Read the model definition and answer for the solid it produces. Units are mm, in the model's axes. A direction names the side the tool comes from. Coordinates: 2 decimals unless noted, no trailing zeros. Loops run counter-clockwise (first coordinate to the right, second up) from the corner with the lowest first, then second, coordinate; pieces in that order, holes last. Notation, with made-up numbers: (51.25, -17) -> (57.25, -17) arc R28 ccw to (57.25, 9) -> close; hole circle Ø1 at (25.5, 11.5). An arc over 180 degrees is marked (long way). Answer as a JSON object with one key per item and string values. Group by question number.
Q1. Each of these flat-tipped pins is pushed along its axis until it touches: P1, Ø4.5, axis at y = -25, z = 48, coming from the -X side; P2, Ø1.9, axis at y = -25, z = 12.5, coming from the +X side; P3, Ø0.8, axis at y = -27, z = 83.5, coming from the -X side; P4, Ø4, axis at x = -14, y = -20.5, coming from the -Z side. Where does it stop, or does it pass through?
Q2. The part is cut by section C-C on x = 40.5. Write down the section's boundary in (y, z).
Q3. Determine the mould class of faces 4 (the flat face through (-10, -24, 70)), 5 (the flat face through (36, -27.495, 49)), 6 (the flat face through (-7, -25, 100)) for opening direction Z: released by +Z, released by -Z, zero draft, split by the parting line, or undercut.
Q4. The part is cut by section B-B on z = 67.5. Write down the section's boundary in (x, y), and give its area (3 significant figures).
Q5. The part is cut by section A-A on x = -2.5. Write down the section's boundary in (y, z), and give its area (3 significant figures).
Q6. Straight lines are drawn through the part: line 1 along Z through (x, y) = (-22.5, -21.75); line 2 along X through (y, z) = (-25.25, 13); line 3 along Y through (x, z) = (44.5, 78). For each, find the intervals that lie inside material, in ascending order. Write a range as [from, to].
Q7. The part is cut by section D-D on z = 38.5. Write down the section's boundary in (x, y), and give its area (3 significant figures).
Q8. For faces 1 (the flat face through (-9, -24, 30)), 2 (the flat face through (-7, -25, 0)), 3 (the flat face through (4.258, -26, 85)), determine the directions among +Z, -Z, +X, -X, +Y, -Y from which every point of the face is accessible in a straight line to the end or side of a thin tool.
from build123d import *

# Parameters (mm, degrees)
BOSS_EXTRUDE1_DEPTH     = 100
CUT_EXTRUDE1_DEPTH      = 24
CUT_EXTRUDE1_DEPTH_BACK = 24
FILLET2_R               = 25
SKETCH4_W               = 13
SKETCH4_H               = 10
CUT_EXTRUDE3_DEPTH      = 23


with BuildPart() as part:
    # Sketch1 → Boss-Extrude1 (new body)
    with BuildSketch(Plane.XY):
        with BuildLine():
            Line((-25.742274507, -27.495485701), (-25.742274507, -25.803839777))
            ThreePointArc((-25.742274507, -25.803839777), (-25.800853151, -25.66241842), (-25.942274507, -25.603839777))
            Line((-25.942274507, -25.603839777), (-26.659431795, -25.603839777))
            ThreePointArc((-26.659431795, -25.603839777), (-26.735968481, -25.588615683), (-26.800853151, -25.545261133))
            Line((-26.800853151, -25.545261133), (-27.683698081, -24.662416203))
            ThreePointArc((-27.683698081, -24.662416203), (-27.72705275, -24.597531247), (-27.742276725, -24.520994228))
            Line((-27.742276725, -24.520994228), (-27.742274507, -23.803840395))
            ThreePointArc((-27.742274507, -23.803840395), (-27.800852932, -23.662418639), (-27.942274507, -23.603839777))
            Line((-27.942274507, -23.603839777), (-28.659430376, -23.603840885))
            ThreePointArc((-28.659430376, -23.603840885), (-28.735967229, -23.588616851), (-28.800852042, -23.545262242))
            Line((-28.800852042, -23.545262242), (-29.683696972, -22.662417311))
            ThreePointArc((-29.683696972, -22.662417311), (-29.727051582, -22.597532499), (-29.742275616, -22.520995646))
            Line((-29.742275616, -22.520995646), (-29.742274507, -21.803839777))
            ThreePointArc((-29.742274507, -21.803839777), (-29.800853256, -21.662418316), (-29.942274803, -21.603839777))
            Line((-29.942274803, -21.603839777), (-30.659430376, -21.603840885))
            ThreePointArc((-30.659430376, -21.603840885), (-30.735967229, -21.588616851), (-30.800852042, -21.545262242))
            Line((-30.800852042, -21.545262242), (-31.683696972, -20.662417311))
            ThreePointArc((-31.683696972, -20.662417311), (-31.727051582, -20.597532499), (-31.742275616, -20.520995646))
            Line((-31.742275616, -20.520995646), (-31.742274507, -19.80383981))
            ThreePointArc((-31.742274507, -19.80383981), (-31.800854095, -19.662417476), (-31.942277212, -19.603839777))
            Line((-31.942277212, -19.603839777), (-32.659432785, -19.603840885))
            ThreePointArc((-32.659432785, -19.603840885), (-32.735969638, -19.588616851), (-32.80085445, -19.545262242))
            Line((-32.80085445, -19.545262242), (-33.683699381, -18.662417311))
            ThreePointArc((-33.683699381, -18.662417311), (-33.727054119, -18.597532189), (-33.742278024, -18.520994974))
            Line((-33.742278024, -18.520994974), (-33.742274507, -17.803842952))
            ThreePointArc((-33.742274507, -17.803842952), (-33.683696986, -17.662419543), (-33.542274507, -17.603839777))
            Line((-33.542274507, -17.603839777), (-23.942274507, -17.603839777))
            ThreePointArc((-23.942274507, -17.603839777), (-23.800853151, -17.66241842), (-23.742274507, -17.803839777))
            Line((-23.742274507, -17.803839777), (-23.742274507, -18.520997064))
            ThreePointArc((-23.742274507, -18.520997064), (-23.727050414, -18.597533751), (-23.683695863, -18.66241842))
            Line((-23.683695863, -18.66241842), (-22.800853151, -19.545261133))
            ThreePointArc((-22.800853151, -19.545261133), (-22.735968481, -19.588615683), (-22.659431795, -19.603839777))
            Line((-22.659431795, -19.603839777), (-21.942274507, -19.603839777))
            ThreePointArc((-21.942274507, -19.603839777), (-21.800853151, -19.66241842), (-21.742274507, -19.803839777))
            Line((-21.742274507, -19.803839777), (-21.742274507, -20.520997064))
            ThreePointArc((-21.742274507, -20.520997064), (-21.727050414, -20.597533751), (-21.683695863, -20.66241842))
            Line((-21.683695863, -20.66241842), (-20.800853151, -21.545261133))
            ThreePointArc((-20.800853151, -21.545261133), (-20.735968481, -21.588615683), (-20.659431795, -21.603839777))
            Line((-20.659431795, -21.603839777), (-19.942274507, -21.603839777))
            ThreePointArc((-19.942274507, -21.603839777), (-19.800853151, -21.66241842), (-19.742274507, -21.803839777))
            Line((-19.742274507, -21.803839777), (-19.742274507, -22.520997064))
            ThreePointArc((-19.742274507, -22.520997064), (-19.727050414, -22.597533751), (-19.683695863, -22.66241842))
            Line((-19.683695863, -22.66241842), (-18.742274507, -23.603839777))
            Line((-18.742274507, -23.603839777), (-17.742274507, -23.603839777))
            Line((-17.742274507, -23.603839777), (59.257725493, -23.603839777))
            Line((59.257725493, -23.603839777), (59.257725493, -27.495485701))
            Line((59.257725493, -27.495485701), (-25.742274507, -27.495485701))
        make_face()
    extrude(amount=BOSS_EXTRUDE1_DEPTH)

    # Sketch2 → Cut-Extrude1 (cut, two sides: drawn at the far end of the back side and taken through both)
    with BuildSketch(Plane(origin=(0, -23.603839777, 0), x_dir=(1, 0, 0), z_dir=(0, 1, 0)).offset(-CUT_EXTRUDE1_DEPTH_BACK)):
        with BuildLine():
            Line((14.257725493, -30), (-42.622702361, -30))
            Line((-42.622702361, -30), (-42.622702361, -70))
            Line((-42.622702361, -70), (14.257725493, -70))
            ThreePointArc((14.257725493, -70), (24.864327211, -65.606601718), (29.257725493, -55))
            Line((29.257725493, -55), (29.257725493, -45))
            ThreePointArc((29.257725493, -45), (24.864327211, -34.393398282), (14.257725493, -30))
        make_face()
    extrude(amount=CUT_EXTRUDE1_DEPTH + CUT_EXTRUDE1_DEPTH_BACK, mode=Mode.SUBTRACT)

    # Fillet2
    fillet2_edges = [part.edges().sort_by_distance(p)[0] for p in [
        (59.257725493, -25.549662739, 100),
        (59.257725493, -25.549662739, 0),
    ]]
    fillet(fillet2_edges, radius=FILLET2_R)

    # Sketch4 → Cut-Extrude3 (cut)
    with BuildSketch(Plane(origin=(0, -23.603839777, 0), x_dir=(1, 0, 0), z_dir=(0, 1, 0))):
        with BuildLine():
            Line((14.257725493, -90), (14.257725493, -80))
            ThreePointArc((14.257725493, -80), (31.935395023, -72.67766953), (39.257725493, -55))
            Line((39.257725493, -55), (49.257725493, -55))
            ThreePointArc((49.257725493, -55), (39.006462834, -79.748737342), (14.257725493, -90))
        make_face()
        with Locations((-2.242274507, -85)):
            Rectangle(SKETCH4_W, SKETCH4_H)
        with BuildLine():
            Line((14.257725493, -20), (14.257725493, -10))
            ThreePointArc((14.257725493, -10), (39.006462834, -20.251262658), (49.257725493, -45))
            Line((49.257725493, -45), (39.257725493, -45))
            ThreePointArc((39.257725493, -45), (31.935395023, -27.32233047), (14.257725493, -20))
        make_face()
        with Locations((-2.242274507, -15)):
            Rectangle(SKETCH4_W, SKETCH4_H)
    extrude(amount=-CUT_EXTRUDE3_DEPTH, mode=Mode.SUBTRACT)


solid = part.part
Final values:
{
 "1": {"P1": "stops at x = 29.26", "P2": "stops at x = 56.43", "P3": "stops at x = -25.74", "P4": "passes through"},
 "2": {"outline": "(-27.5, 0.79) -> (-23.6, 0.79) -> (-23.6, 21.84) -> (-27.5, 21.84) -> close; (-27.5, 45) -> (-23.6, 45) -> (-23.6, 55) -> (-27.5, 55) -> close; (-27.5, 78.16) -> (-23.6, 78.16) -> (-23.6, 99.21) -> (-27.5, 99.21) -> close"},
 "3": {"face 4": "undercut", "face 5": "zero draft", "face 6": "released by +Z"},
 "4": {"outline": "(22.55, -27.5) -> (35.91, -27.5) -> (35.91, -23.6) -> (22.55, -23.6) -> close; (46.95, -27.5) -> (59.26, -27.5) -> (59.26, -23.6) -> (46.95, -23.6) -> close", "area": "99.9 mm2"},
 "5": {"outline": "(-27.5, 0) -> (-23.6, 0) -> (-23.6, 10) -> (-27.5, 10) -> close; (-27.5, 20) -> (-23.6, 20) -> (-23.6, 30) -> (-27.5, 30) -> close; (-27.5, 70) -> (-23.6, 70) -> (-23.6, 80) -> (-27.5, 80) -> close; (-27.5, 90) -> (-23.6, 90) -> (-23.6, 100) -> (-27.5, 100) -> close", "area": "156 mm2"},
 "6": {"line 1": "z = [0, 30], [70, 100]", "line 2": "x = [-27.1, -8.74], [4.26, 14.26], [28.44, 56.19]", "line 3": "y = [-27.5, -23.6]"},
 "7": {"outline": "(27.78, -27.5) -> (38.4, -27.5) -> (38.4, -23.6) -> (27.78, -23.6) -> close; (48.65, -27.5) -> (59.26, -27.5) -> (59.26, -23.6) -> (48.65, -23.6) -> close", "area": "82.6 mm2"},
 "8": {"face 1": "-X, +Y, -Y", "face 2": "-Z, +X, -X, +Y, -Y", "face 3": "+Y, -Y"}
}
